from build123d import *

# Parameters (mm, degrees)
F1_DEPTH = 127


with BuildPart() as f1:
    # F0 (on Right) → F1 (new body)
    with BuildSketch(Plane.YZ):
        with BuildLine():
            Line((-25.4, 76.2), (-25.4, 2.54))
            Line((-25.4, 2.54), (-20.32, 2.54))
            Line((-20.32, 2.54), (-20.32, 76.2))
            ThreePointArc((-20.32, 76.2), (-21.063949, 77.996051), (-22.86, 78.74))
            ThreePointArc((-22.86, 78.74), (-24.656051, 77.996051), (-25.4, 76.2))
        make_face()
        Polygon((-20.32, 2.54), (-25.4, 2.54), (-25.4, -2.54), (25.4, -2.54), (25.4, 2.54), (20.32, 2.54), (2.798074, 2.54), (-2.281926, 2.54), align=None)
        with BuildLine():
            Line((-2.281926, 65.054222), (-2.281926, 2.54))
            Line((-2.281926, 2.54), (2.798074, 2.54))
            Line((2.798074, 2.54), (2.798074, 65.054222))
            ThreePointArc((2.798074, 65.054222), (2.054126, 66.850273), (0.258074, 67.594222))
            ThreePointArc((0.258074, 67.594222), (-1.537977, 66.850273), (-2.281926, 65.054222))
        make_face()
        with BuildLine():
            Line((20.32, 2.54), (25.4, 2.54))
            Line((25.4, 2.54), (25.4, 50.8))
            ThreePointArc((25.4, 50.8), (24.656051, 52.596051), (22.86, 53.34))
            ThreePointArc((22.86, 53.34), (21.063949, 52.596051), (20.32, 50.8))
            Line((20.32, 50.8), (20.32, 2.54))
        make_face()
    extrude(amount=F1_DEPTH)


solid = f1.part
Geometry check sheet. Reference: the model listing, model coordinates, mm. A direction names the side the tool comes from. Give positions to 0.01 mm unless a question says otherwise; leave off trailing zeros. Loops run counter-clockwise (first coordinate to the right, second up) from the corner with the lowest first, then second, coordinate; pieces in that order, holes last. Notation, with made-up numbers: (-20.5, -9) -> (33.5, -9) arc R26 cw to (33.5, 26) -> close; hole circle Ø8 at (-20, -30). An arc over 180 degrees is marked (long way). Answer in a Markdown table with one row per item. Add a question column.
1) Cross-section at D-D on y = 5. Record the boundary of the cut face in (x, z).
2) Material ranges on probe 1 along Y at (x, z) = (91, 5.5); probe 2 along Y at (x, z) = (79.5, 68.5); probe 3 along Y at (x, z) = (16.5, 67), recorded low to high. Write a range as from..to.
3) Cross-section at A-A on z = 55.5. Record the boundary of the cut face in (x, y), and give its area (3 significant figures).
4) Cross-section at B-B on z = 37.5. Record the boundary of the cut face in (x, y), and give its area (3 significant figures).
5) Set-up check for faces 5 (the face through (63, 20.32, 27)), 6 (the face through (63, -25.4, 37)): record each of +Z, -Z, +X, -X, +Y, -Y from which the full face is reachable in a straight line by a thin tool's end or side.
6) Cross-section at C-C on x = 56.5. Record the boundary of the cut face in (y, z), and give its area (3 significant figures).
7) Gauge pin test, flat ends, axial feed: P1, Ø5, axis at x = 74, y = 13, coming from the +Z side; P2, Ø6, axis at x = 114, y = -5, coming from the +Z side; P3, Ø12, axis at y = -19, z = 13, coming from the +X side; P4, Ø5, axis at x = 78, y = 2.5, coming from the +Z side. Record the tip position at first contact, or that the pin passes through.
8) Draft check along Y on faces 1 (the face through (63, -11, 2.54)), 2 (the face through (63, 25.4, 24)), 3 (the face through (127, 0, 26)), 4 (the face through (63, 2.798, 33)). Enter one of: pulls with the +Y half, pulls with the -Y half, needs draft (parallel to the pull), parting line crosses it, or undercut.
Outcome:
| question | item | result |
|---|---|---|
| 1 | outline | (0, -2.54) -> (127, -2.54) -> (127, 2.54) -> (0, 2.54) -> close |
| 2 | probe 1 | y = -25.4..-20.32, -2.28..2.8, 20.32..25.4 |
| 2 | probe 2 | y = -25.4..-20.32 |
| 2 | probe 3 | y = -25.4..-20.32, -1.37..1.89 |
| 3 | outline | (0, -25.4) -> (127, -25.4) -> (127, -20.32) -> (0, -20.32) -> close; (0, -2.28) -> (127, -2.28) -> (127, 2.8) -> (0, 2.8) -> close |
| 3 | area | 1,290 mm^2 |
| 4 | outline | (0, -25.4) -> (127, -25.4) -> (127, -20.32) -> (0, -20.32) -> close; (0, -2.28) -> (127, -2.28) -> (127, 2.8) -> (0, 2.8) -> close; (0, 20.32) -> (127, 20.32) -> (127, 25.4) -> (0, 25.4) -> close |
| 4 | area | 1,940 mm^2 |
| 5 | face 5 | +Z, +X, -X |
| 5 | face 6 | +Z, -Z, +X, -X, -Y |
| 6 | outline | (-25.4, -2.54) -> (25.4, -2.54) -> (25.4, 50.8) arc R2.54 ccw to (22.86, 53.34) arc R2.54 ccw to (20.32, 50.8) -> (20.32, 2.54) -> (2.8, 2.54) -> (2.8, 65.05) arc R2.54 ccw to (0.26, 67.59) arc R2.54 ccw to (-2.28, 65.05) -> (-2.28, 2.54) -> (-20.32, 2.54) -> (-20.32, 76.2) arc R2.54 ccw to (-22.86, 78.74) arc R2.54 ccw to (-25.4, 76.2) -> close |
| 6 | area | 1,230 mm^2 |
| 7 | P1 | stops at z = 2.54 |
| 7 | P2 | stops at z = 66.22 |
| 7 | P3 | stops at x = 127 |
| 7 | P4 | stops at z = 67.59 |
| 8 | face 1 | undercut |
| 8 | face 2 | pulls with the +Y half |
| 8 | face 3 | needs draft |
| 8 | face 4 | undercut |
